from build123d import *

# Parameters (mm, degrees)
SKETCH1_R           = 4.5
SKETCH1_R_2         = 1.7
BOSS_EXTRUDE1_DEPTH = 1.5
BOSS_EXTRUDE2_DEPTH = 5
SKETCH4_R           = 0.5
CUT_EXTRUDE1_DEPTH  = 14.756816492
FILLET1_R           = 1.5


with BuildPart() as part:
    # Sketch1 → Boss-Extrude1 (new body)
    with BuildSketch(Plane(origin=(0, 0, 0), x_dir=(1, 0, 0), z_dir=(0, 1, 0))):
        with Locations(Location((0, 0, 0), (0, 0, 270))):
            Circle(SKETCH1_R)
        with Locations(Location((0, 0, 0), (0, 0, 270))):
            Circle(SKETCH1_R_2, mode=Mode.SUBTRACT)
    extrude(amount=BOSS_EXTRUDE1_DEPTH)

    # Sketch3 → Boss-Extrude2 (add)
    with BuildSketch(Plane(origin=(0, 0, 0), x_dir=(1, 0, 0), z_dir=(0, 1, 0))):
        with BuildLine():
            Line((-1.5, -4.242640687), (-1.5, -6))
            Line((-1.5, -6), (1.5, -6))
            Line((1.5, -6), (1.5, -4.242640687))
            ThreePointArc((1.5, -4.242640687), (0, -4.5), (-1.5, -4.242640687))
        make_face()
        with BuildLine():
            Line((-1.5, 6), (1.5, 6))
            Line((1.5, 6), (1.5, 4.242640687))
            ThreePointArc((1.5, 4.242640687), (0, 4.5), (-1.5, 4.242640687))
            Line((-1.5, 4.242640687), (-1.5, 6))
        make_face()
    extrude(amount=BOSS_EXTRUDE2_DEPTH)

    # Sketch4 → Cut-Extrude1 (cut, through all)
    with BuildSketch(Plane.XY.offset(6)):
        with Locations((0, 3.5)):
            Circle(SKETCH4_R)
    extrude(amount=-CUT_EXTRUDE1_DEPTH, mode=Mode.SUBTRACT)

    # Fillet1
    fillet1_edges = [part.edges().sort_by_distance(p)[0] for p in [
        (1.5, 5, 5.121320344),
        (-1.5, 5, 5.121320344),
        (1.5, 5, -5.121320344),
        (-1.5, 5, -5.121320344),
    ]]
    fillet(fillet1_edges, radius=FILLET1_R - 0.0001)  # a hair under: the kernel refuses the full size


solid = part.part
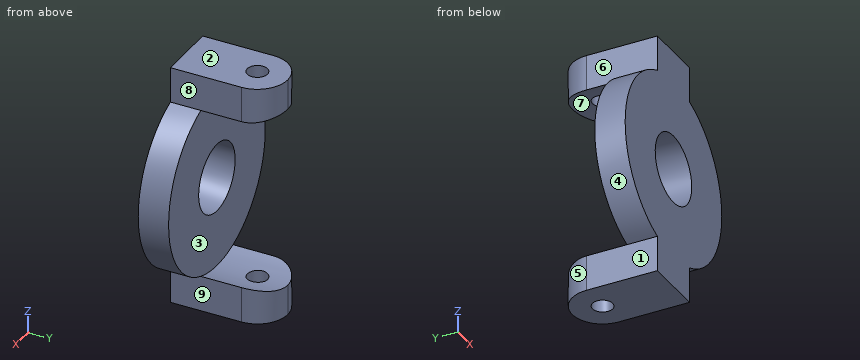
Source: CAD feature listing. Evaluate the final solid. Frame: model axes, mm. Face numbers are marked on the shaded views. A direction names the side the tool comes from. Round coordinates to 2 decimals unless told otherwise and drop trailing zeros. Loops run counter-clockwise (first coordinate to the right, second up) from the corner with the lowest first, then second, coordinate; pieces in that order, holes last. Notation, with made-up numbers: (82, 12.5) - (89, 12.5) arc R14 cw to (89, 18.5) - close; hole circle Ø3 at (85, -34). An arc over 180 degrees is marked (long way). Write item = value, one per line. Start each with the question number.
Item 1: Section query C-C on x = 1.25. Output: boundary loops of the cut face in (y, z).
Item 2: Reachability of the marked faces 5, 6, 7, 8 and 9 from +Z, -Z, +X, -X, +Y, -Y: full face, straight path, thin tool, end or side. Return the list, or none.
Item 3: Section query A-A on y = 1.25. Output: boundary loops of the cut face in (x, z), plus the area to 3 significant figures.
Item 4: Material intervals for line 1 (X direction, y = 3.5, z = 5.1); line 2 (Y direction, x = 0, z = -4.9); line 3 (Y direction, x = 0.5, z = -2.5), sorted ascending.
Item 5: Section query D-D on y = 4.35. Output: boundary loops of the cut face in (x, z), plus the area to 3 significant figures.
Item 6: Section query B-B on z = 0. Output: boundary loops of the cut face in (x, y).
Item 7: First-contact query: pin 1 Ø1.4 at (y, z) = (2, -5) entering from +X; pin 2 Ø4.5 at (x, z) = (2, 2) entering from +Y; pin 3 Ø2 at (x, y) = (3, 1.5) entering from +Z; pin 4 Ø4 at (x, z) = (0, 0) entering from -Y. Flat tips, straight axial feed; report the tip coordinate or a pass-through.
Item 8: Mould query, pull axis Z, two halves, no side actions, for the marked faces 1, 2, 3 and 4. Classes: released by +Z, released by -Z, zero draft, split by the parting line, or undercut.
Results list:
q1.outline = (0, -6) - (4.33, -6) - (4.33, -4.32) - (1.5, -4.32) - (1.5, -1.15) - (0, -1.15) - close; (0, 1.15) - (1.5, 1.15) - (1.5, 4.32) - (4.33, 4.32) - (4.33, 6) - (0, 6) - close
q2.face_5 = +Z, -Z, -X, +Y
q2.face_6 = +Z, -X, +Y, -Y
q2.face_7 = +Y
q2.face_8 = +Z, +X, +Y, -Y
q2.face_9 = -Z, +X, +Y, -Y
q3.outline = (-1.5, -6) - (1.5, -6) - (1.5, -4.24) arc R4.5 ccw to (1.5, 4.24) - (1.5, 6) - (-1.5, 6) - (-1.5, 4.24) arc R4.5 ccw to (-1.5, -4.24) - close; hole circle Ø3.4 at (0, 0)
q3.area = 64.0 mm²
q4.line_1 = -1.5 to -0.5, 0.5 to 1.5
q4.line_2 = 0 to 3, 4 to 5
q4.line_3 = 0 to 1.5
q5.outline = (-1.24, -6) - (1.24, -6) - (1.24, -4.33) arc R4.5 cw to (-1.24, -4.33) - close; (-1.24, 4.33) arc R4.5 cw to (1.24, 4.33) - (1.24, 6) - (-1.24, 6) - close
q5.area = 7.70 mm²
q6.outline = (-4.5, 0) - (-1.7, 0) - (-1.7, 1.5) - (-4.5, 1.5) - close; (1.7, 0) - (4.5, 0) - (4.5, 1.5) - (1.7, 1.5) - close
q7.pin_1 = 1.5
q7.pin_2 = 1.5
q7.pin_3 = 4.03
q7.pin_4 = 0
q8.face_1 = zero draft
q8.face_2 = released by +Z
q8.face_3 = undercut
q8.face_4 = split by the parting line
